```python
from build123d import *

# Parameters (mm, degrees)
Y_KSEKLIK_EKSTR_ZYON1_DEPTH = 372
KES_EKSTR_ZYON1_DEPTH       = 41
KES_EKSTR_ZYON1_DEPTH_BACK  = 43
KES_EKSTR_ZYON2_DEPTH       = 72
KES_EKSTR_ZYON2_DEPTH_BACK  = 61


with BuildPart() as part:
    # Çizim1 → Yükseklik-Ekstrüzyon1 (new body)
    with BuildSketch(Plane.XY):
        with BuildLine():
            Line((-16, 20), (16, 20))
            ThreePointArc((16, 20), (18.828427125, 18.828427125), (20, 16))
            Line((20, 16), (20, -16))
            ThreePointArc((20, -16), (18.828427125, -18.828427125), (16, -20))
            Line((16, -20), (-16, -20))
            ThreePointArc((-16, -20), (-18.828427125, -18.828427125), (-20, -16))
            Line((-20, -16), (-20, 16))
            ThreePointArc((-20, 16), (-18.828427125, 18.828427125), (-16, 20))
        make_face()
        with BuildLine():
            Line((-18, 16), (-18, -16))
            ThreePointArc((-18, -16), (-17.414213562, -17.414213562), (-16, -18))
            Line((-16, -18), (16, -18))
            ThreePointArc((16, -18), (17.414213562, -17.414213562), (18, -16))
            Line((18, -16), (18, 16))
            ThreePointArc((18, 16), (17.414213562, 17.414213562), (16, 18))
            Line((16, 18), (-16, 18))
            ThreePointArc((-16, 18), (-17.414213562, 17.414213562), (-18, 16))
        make_face(mode=Mode.SUBTRACT)
    extrude(amount=Y_KSEKLIK_EKSTR_ZYON1_DEPTH)

    # Çizim3 → Kes-Ekstrüzyon1 (cut, two sides: drawn at the far end of the back side and taken through both)
    with BuildSketch(Plane(origin=(0, 0, 0), x_dir=(0, 0, -1), z_dir=(1, 0, 0)).offset(-KES_EKSTR_ZYON1_DEPTH_BACK)):
        Polygon((-372, 20), (-332, -20), (-372, -20), align=None)
    extrude(amount=KES_EKSTR_ZYON1_DEPTH + KES_EKSTR_ZYON1_DEPTH_BACK, mode=Mode.SUBTRACT)

    # Çizim5 → Kes-Ekstrüzyon2 (cut, two sides: drawn at the far end of the back side and taken through both)
    with BuildSketch(Plane(origin=(0, 0, 0), x_dir=(1, 0, 0), z_dir=(0, 1, 0)).offset(-KES_EKSTR_ZYON2_DEPTH_BACK)):
        Polygon((20, 0), (-20, -40), (-20, 0), align=None)
    extrude(amount=KES_EKSTR_ZYON2_DEPTH + KES_EKSTR_ZYON2_DEPTH_BACK, mode=Mode.SUBTRACT)


solid = part.part
```
Input: part model. Units: mm. Frame: model coordinates. A direction names the side the tool comes from. Give positions to 0.01 mm unless a question says otherwise; leave off trailing zeros. Order: outer loops, then holes, each group sorted by start corner. A loop starts at its lowest first (then second) coordinate and runs counter-clockwise, first axis right, second up.
1. Section A-A on x = 6. Return the cut outline in (y, z), and give its area (3 significant figures).
Derived:
outline: (-20, 14) - (-18, 14) - (-18, 334) - (-20, 332) - close; (18, 14) - (20, 14) - (20, 372) - (18, 370) - close
area: 1,350 mm2
2. Pin query (flat end, axial travel): pin 1 (8 mm diameter, centred on x = 4.5, y = -13.5, fed in from +Z). Return the tip coordinate at first contact, or that it passes through.
Derived:
pin 1: passes through
3. Mould query, pull axis Z, two halves, no side actions, for faces 3 (the flat face through (0, -18, 167)), 4 (the flat face through (19, 2, 354)), 5 (the flat face through (2, 19, 18)). Classes: released by +Z, released by -Z, zero draft, split by the parting line, or undercut.
Derived:
face 3: zero draft
face 4: released by +Z
face 5: released by -Z
4. Section C-C on z = 124.5. Return the cut outline in (x, y), and give its area (3 significant figures).
Derived:
outline: (-20, -16) arc R4 ccw to (-16, -20) - (16, -20) arc R4 ccw to (20, -16) - (20, 16) arc R4 ccw to (16, 20) - (-16, 20) arc R4 ccw to (-20, 16) - close; hole (-18, -16) arc R2 ccw to (-16, -18) - (16, -18) arc R2 ccw to (18, -16) - (18, 16) arc R2 ccw to (16, 18) - (-16, 18) arc R2 ccw to (-18, 16) - close
area: 294 mm2
5. Section D-D on z = 339.5. Return the cut outline in (x, y).
Derived:
outline: (-20, -12.5) - (-18, -12.5) - (-18, 16) arc R2 cw to (-16, 18) - (16, 18) arc R2 cw to (18, 16) - (18, -12.5) - (20, -12.5) - (20, 16) arc R4 ccw to (16, 20) - (-16, 20) arc R4 ccw to (-20, 16) - close
6. Reachability of faces 1 (the flat face through (20, 0, 181)), 2 (the flat face through (0, 18, 184)) from +Z, -Z, +X, -X, +Y, -Y: full face, straight path, thin tool, end or side. Return the list, or none.
Derived:
face 1: +Z, -Z, +X, +Y, -Y
face 2: +Z, -Z
7. Section B-B on y = 10. Return the cut outline in (x, z), and give its area (3 significant figures).
Derived:
outline: (-20, 40) - (-18, 38) - (-18, 362) - (-20, 362) - close; (18, 2) - (20, 0) - (20, 362) - (18, 362) - close
area: 1,370 mm2
8. Material intervals for L1, parallel to X at y = -10.5, z = 258; L2, parallel to X at y = -17, z = 79, sorted ascending.
Derived:
L1: x = -20 to -18, 18 to 20
L2: x = -19.87 to -17.73, 17.73 to 19.87
